Verification items for the finished model (mm, model axes). Give positions to 0.01 mm unless a question says otherwise; leave off trailing zeros. Write each loop counter-clockwise with the first axis right and the second up, starting at its lowest first coordinate (ties: lowest second). Pieces come first, ordered by that corner, then holes. Notation, with made-up numbers: M -7.75,32.5 L 1.25,32.5 A11 ccw 1.25,50.5 Z; hole C 65.25,-29 d4. An arc over 180 degrees is marked long. Write item = value, one per line.
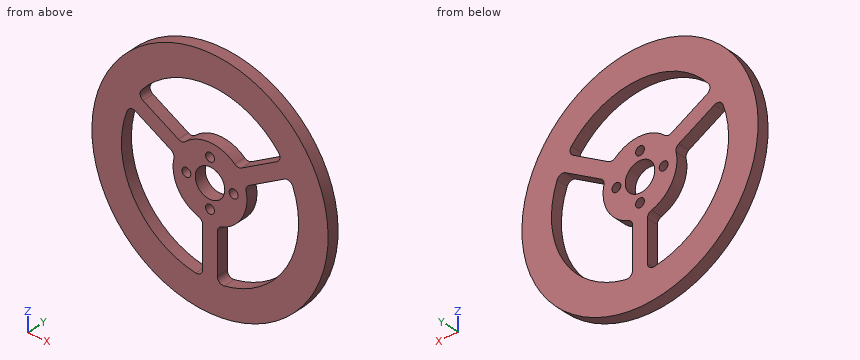
from build123d import *

# Parameters (mm, degrees)
ESBO_O1_R                = 40
ESBO_O1_R_2              = 1.5
ESBO_O1_R_3              = 5
RESSALTO_EXTRUS_O1_DEPTH = 4


with BuildPart() as part:
    # Esboço1 → Ressalto-extrusão1 (new body)
    with BuildSketch(Plane(origin=(0, 4, 0), x_dir=(1, 0, 0), z_dir=(0, 1, 0))):
        with Locations(Location((0, 0, 0), (0, 0, 90))):
            Circle(ESBO_O1_R)
        with Locations(Location((-8, 0, 0), (0, 0, 90))):
            Circle(ESBO_O1_R_2, mode=Mode.SUBTRACT)
        with Locations(Location((0, -8, 0), (0, 0, 90))):
            Circle(ESBO_O1_R_2, mode=Mode.SUBTRACT)
        with Locations(Location((8, 0, 0), (0, 0, 90))):
            Circle(ESBO_O1_R_2, mode=Mode.SUBTRACT)
        with Locations(Location((0, 8, 0), (0, 0, 90))):
            Circle(ESBO_O1_R_2, mode=Mode.SUBTRACT)
        with Locations(Location((0, 0, 0), (0, 0, 90))):
            Circle(ESBO_O1_R_3, mode=Mode.SUBTRACT)
        with BuildLine():
            Line((-2.5, 27.636027211), (-2.5, 13.784048752))
            ThreePointArc((-2.5, 13.784048752), (-2.881145573, 12.609608313), (-3.879310345, 11.882800648))
            ThreePointArc((-3.879310345, 11.882800648), (-10.825317547, 6.25), (-12.230462402, -2.581819016))
            ThreePointArc((-12.230462402, -2.581819016), (-12.360813917, -3.809658898), (-13.187336386, -4.726960867))
            Line((-13.187336386, -4.726960867), (-25.183501624, -11.652950096))
            ThreePointArc((-25.183501624, -11.652950096), (-26.855199812, -11.804730901), (-28.05375174, -10.629534952))
            ThreePointArc((-28.05375174, -10.629534952), (-25.980762114, 15), (-4.821428571, 29.610029155))
            ThreePointArc((-4.821428571, 29.610029155), (-3.204403061, 29.159650711), (-2.5, 27.636027211))
        make_face(mode=Mode.SUBTRACT)
        with BuildLine():
            Line((25.183501624, -11.652950096), (13.187336386, -4.726960867))
            ThreePointArc((13.187336386, -4.726960867), (12.360813917, -3.809658898), (12.230462402, -2.581819016))
            ThreePointArc((12.230462402, -2.581819016), (10.825317547, 6.25), (3.879310345, 11.882800648))
            ThreePointArc((3.879310345, 11.882800648), (2.881145573, 12.609608313), (2.5, 13.784048752))
            Line((2.5, 13.784048752), (2.5, 27.636027211))
            ThreePointArc((2.5, 27.636027211), (3.204403061, 29.159650711), (4.821428571, 29.610029155))
            ThreePointArc((4.821428571, 29.610029155), (25.980762114, 15), (28.05375174, -10.629534952))
            ThreePointArc((28.05375174, -10.629534952), (26.855199812, -11.804730901), (25.183501624, -11.652950096))
        make_face(mode=Mode.SUBTRACT)
        with BuildLine():
            Line((10.687336386, -9.057087886), (22.683501624, -15.983077115))
            ThreePointArc((22.683501624, -15.983077115), (23.650796751, -17.35491981), (23.232323169, -18.980494203))
            ThreePointArc((23.232323169, -18.980494203), (0, -30), (-23.232323169, -18.980494203))
            ThreePointArc((-23.232323169, -18.980494203), (-23.650796751, -17.35491981), (-22.683501624, -15.983077115))
            Line((-22.683501624, -15.983077115), (-10.687336386, -9.057087886))
            ThreePointArc((-10.687336386, -9.057087886), (-9.479668344, -8.799949415), (-8.351152057, -9.300981632))
            ThreePointArc((-8.351152057, -9.300981632), (0, -12.5), (8.351152057, -9.300981632))
            ThreePointArc((8.351152057, -9.300981632), (9.479668344, -8.799949415), (10.687336386, -9.057087886))
        make_face(mode=Mode.SUBTRACT)
    extrude(amount=-RESSALTO_EXTRUS_O1_DEPTH)


solid = part.part
1) Depth check by flat-ended pin: P1, Ø4, axis at x = 8, z = 0, coming from the -Y side; P2, Ø2, axis at y = 2, z = -20, coming from the -X side; P3, Ø1.5, axis at y = 1, z = 0, coming from the -X side; P4, Ø2, axis at y = 2, z = -21.5, coming from the +X side. Enter the tip coordinate at first touch or a pass-through.
From the geometry:
P1 = 0
P2 = -35.2
P3 = -40
P4 = 34.35
2) Cross-section at D-D on x = 27. Record the boundary of the cut face in (y, z), plus the area to 3 significant figures.
From the geometry:
outline = M 0,-29.51 L 4,-29.51 L 4,-13.08 L 0,-13.08 Z; M 0,11.75 L 4,11.75 L 4,29.51 L 0,29.51 Z
area = 137 mm^2
3) Cross-section at B-B on z = 0. Record the boundary of the cut face in (x, y).
From the geometry:
outline = M -40,0 L -30,0 L -30,4 L -40,4 Z; M -12.5,0 L -9.5,0 L -9.5,4 L -12.5,4 Z; M -6.5,0 L -5,0 L -5,4 L -6.5,4 Z; M 5,0 L 6.5,0 L 6.5,4 L 5,4 Z; M 9.5,0 L 12.5,0 L 12.5,4 L 9.5,4 Z; M 30,0 L 40,0 L 40,4 L 30,4 Z
4) Cross-section at C-C on z = 23. Record the boundary of the cut face in (x, y).
From the geometry:
outline = M -32.73,0 L -19.26,0 L -19.26,4 L -32.73,4 Z; M 19.26,0 L 32.73,0 L 32.73,4 L 19.26,4 Z
5) Material ranges on probe 1 along X at (y, z) = (1.75, 0); probe 2 along Z at (x, y) = (-11.5, 2.95); probe 3 along Z at (x, y) = (8, 1.5), recorded low to high. Write a range as from..to.
From the geometry:
probe_1 = -40..-30, -12.5..-9.5, -6.5..-5, 5..6.5, 9.5..12.5, 30..40
probe_2 = -38.31..-27.71, -4.9..9.53, 27.71..38.31
probe_3 = -39.19..-28.91, -9.6..-1.5, 1.5..9.6, 28.91..39.19
6) Cross-section at A-A on x = 0. Record the boundary of the cut face in (y, z), plus the area to 3 significant figures.
From the geometry:
outline = M 0,-40 L 4,-40 L 4,-9.5 L 0,-9.5 Z; M 0,-6.5 L 4,-6.5 L 4,-5 L 0,-5 Z; M 0,5 L 4,5 L 4,6.5 L 0,6.5 Z; M 0,9.5 L 4,9.5 L 4,12.5 L 0,12.5 Z; M 0,30 L 4,30 L 4,40 L 0,40 Z
area = 186 mm^2
